from build123d import *

# Parameters (mm, degrees)
SKETCH1_W             = 85
SKETCH1_H             = 74
BOSS_EXTRUDE1_DEPTH   = 9.525
M8_CLEARANCE_HOLE1_D  = 9
M6X1_0_TAPPED_HOLE1_D = 5
M3X0_5_TAPPED_HOLE1_D = 2.5
CHAMFER1_SIZE         = 1


with BuildPart() as part:
    # Sketch1 → Boss-Extrude1 (new body)
    with BuildSketch(Plane(origin=(0, 0, 0), x_dir=(1, 0, 0), z_dir=(0, 1, 0))):
        Rectangle(SKETCH1_W, SKETCH1_H)
    extrude(amount=BOSS_EXTRUDE1_DEPTH)

    # M8 Clearance Hole1 (through all)
    with Locations(Plane(origin=(0, 9.525, 0), x_dir=(1, 0, 0), z_dir=(0, 1, 0))):
        with Locations((-32.5, 20), (32.5, 20), (32.5, -20), (-32.5, -20)):
            Hole(M8_CLEARANCE_HOLE1_D / 2)

    # M6x1.0 Tapped Hole1 (through all)
    with Locations(Plane(origin=(0, 9.525, 0), x_dir=(1, 0, 0), z_dir=(0, 1, 0))):
        with Locations((0, 27), (15, 27), (15, -27), (0, -27)):
            Hole(M6X1_0_TAPPED_HOLE1_D / 2)

    # M3x0.5 Tapped Hole1 (through all)
    with Locations(Plane(origin=(0, 9.525, 0), x_dir=(1, 0, 0), z_dir=(0, 1, 0))):
        with Locations((-29.5, 33), (-10.5, 33)):
            Hole(M3X0_5_TAPPED_HOLE1_D / 2)

    # Chamfer1
    chamfer1_edges = [part.edges().sort_by_distance(p)[0] for p in [
        (42.5, 4.7625, 37),
        (-42.5, 4.7625, 37),
        (-42.5, 4.7625, -37),
        (42.5, 4.7625, -37),
    ]]
    chamfer(chamfer1_edges, length=CHAMFER1_SIZE)


solid = part.part
Source: CAD feature listing. Evaluate the final solid. Frame: model axes, mm. Coordinates: 2 decimals unless noted, no trailing zeros. Loops run counter-clockwise (first coordinate to the right, second up) from the corner with the lowest first, then second, coordinate; pieces in that order, holes last. Notation, with made-up numbers: M 63,-15.5 L 112,-15.5 A21 cw 112,-11.5 Z; hole C 18,40.25 d3. An arc over 180 degrees is marked long. Answer in a Markdown table with one row per item.
Q1. Section C-C on x = -10.5. Return the cut outline in (y, z) (3 decimals).
Answers below:
| item | result |
|---|---|
| outline | M 0,-37 L 9.525,-37 L 9.525,-34.25 L 0,-34.25 Z; M 0,-31.75 L 9.525,-31.75 L 9.525,37 L 0,37 Z |
Q2. Ray query, probe 1 along X at (y, z) = (7, -33); probe 2 along Z at (x, y) = (-32.5, 3); probe 3 along X at (y, z) = (2.5, -27). Return the intervals inside material, ascending. Write a range as from..to.
Answers below:
| item | result |
|---|---|
| probe 1 | x = -42.5..-30.75, -28.25..-11.75, -9.25..42.5 |
| probe 2 | z = -37..-24.5, -15.5..15.5, 24.5..37 |
| probe 3 | x = -42.5..-2.5, 2.5..12.5, 17.5..42.5 |
Q3. First-contact query: pin 1 (7 mm diameter, centred on x = 32.5, z = -20, fed in from -Y) (3 decimals). Flat tip, straight axial feed; report the tip coordinate or a pass-through.
Answers below:
| item | result |
|---|---|
| pin 1 | passes through |
Q4. Draft query along X for faces 1 (the flat face through (-42.5, 5, 1)), 2 (the flat face through (42.5, 5, 1)), 3 (the flat face through (-1, 0, -1)), 4 (the cylindrical face through (30.081, 4.696, -23.794)). Return one class per face: pulls with the +X half, pulls with the -X half, needs draft (parallel to the pull), parting line crosses it, or undercut.
Answers below:
| item | result |
|---|---|
| face 1 | pulls with the -X half |
| face 2 | pulls with the +X half |
| face 3 | needs draft |
| face 4 | undercut |
Q5. Section A-A on x = 32.5. Return the cut outline in (y, z) (3 decimals).
Answers below:
| item | result |
|---|---|
| outline | M 0,-37 L 9.525,-37 L 9.525,-24.5 L 0,-24.5 Z; M 0,-15.5 L 9.525,-15.5 L 9.525,15.5 L 0,15.5 Z; M 0,24.5 L 9.525,24.5 L 9.525,37 L 0,37 Z |
Q6. Section D-D on y = 5.75. State how many separate pieces and enclosed holes the cut face has, plus the area to 3 significant figures.
Answers below:
| item | result |
|---|---|
| separate pieces | 1 |
| enclosed holes | 10 |
| area | 5,950 mm^2 |
Q7. Section B-B on z = 27. Return the cut outline in (x, y) (3 decimals).
Answers below:
| item | result |
|---|---|
| outline | M -42.5,0 L -2.5,0 L -2.5,9.525 L -42.5,9.525 Z; M 2.5,0 L 12.5,0 L 12.5,9.525 L 2.5,9.525 Z; M 17.5,0 L 42.5,0 L 42.5,9.525 L 17.5,9.525 Z |
